The model under review builds one solid part; all positions refer to its coordinate system, in mm. A direction names the side the tool comes from. Coordinates: 2 decimals unless noted, no trailing zeros. Order: outer loops, then holes, each group sorted by start corner. A loop starts at its lowest first (then second) coordinate and runs counter-clockwise, first axis right, second up.
Autodesk Fusion 360 part; units mm, degrees
sketch "Sketch1" plane through (0, 0, 0) normal (0, 1, 0) x (1, 0, 0)
  line L0 (10, 0) -> (76.2, 0)
  line L1 (86.2, 10) -> (86.2, 44.61)
  line L2 (76.2, 54.61) -> (10, 54.61)
  line L3 (0, 44.61) -> (0, 10)
  circle A0 centre (14.6, 51.435) radius 1.6
  circle A1 centre (14.6, 3.175) radius 1.6
  circle A2 centre (80.64, 48.26) radius 1.6
  circle A3 centre (80.64, 6.35) radius 1.6
  arc A4 (0, 10) -> (10, 0) centre (10, 10) ccw
  arc A5 (10, 54.61) -> (0, 44.61) centre (10, 44.61) ccw
  arc A6 (86.2, 44.61) -> (76.2, 54.61) centre (76.2, 44.61) ccw
  arc A7 (76.2, 0) -> (86.2, 10) centre (76.2, 10) ccw
  dimension "d1" = 86.2
  dimension "d2" = 54.61
  dimension "d3" = 3.2
  dimension "d4" = 14.6
  dimension "d5" = 3.175
  dimension "d6" = 48.26
  dimension "d8" = 41.91
  dimension "d10" = 6.35
  dimension "d11" = 65.9
  dimension "d12" = 66.04
  dimension "d13" = 10
  dimension "d36" = 3.11
extrude "Extrude1" add sketch "Sketch1" along normal blind 1.6
sketch "Sketch2" plane through (0, 1.6, 0) normal (0, 1, 0) x (-1, 0, 0)
  circle A0 centre (-14.6, -3.175) radius 1.6
  circle A1 centre (-80.64, -6.35) radius 1.6
  circle A2 centre (-14.6, -51.435) radius 1.6
  circle A3 centre (-80.64, -48.26) radius 1.6
  arc A4 (-76.2, 0) -> (-86.2, -10) centre (-76.2, -10) ccw
  line L0 (-86.2, -10) -> (-86.2, -44.61)
  arc A5 (-86.2, -44.61) -> (-76.2, -54.61) centre (-76.2, -44.61) ccw
  line L1 (-76.2, -54.61) -> (-10, -54.61)
  arc A6 (-10, -54.61) -> (0, -44.61) centre (-10, -44.61) ccw
  line L2 (0, -44.61) -> (0, -10)
  arc A7 (0, -10) -> (-10, 0) centre (-10, -10) ccw
  line L3 (-10, 0) -> (-76.2, 0)
  line L4 (-18.553, -6) -> (-77.553, -6)
  line L5 (-77.553, -6) -> (-77.553, -1)
  line L6 (-77.553, -1) -> (-18.553, -1)
  line L7 (-18.553, -1) -> (-18.553, -6)
  line L8 (-18.553, -53.61) -> (-77.553, -53.61)
  line L9 (-77.553, -53.61) -> (-77.553, -48.61)
  line L10 (-77.553, -48.61) -> (-18.553, -48.61)
  line L11 (-18.553, -48.61) -> (-18.553, -53.61)
  dimension "d16" = 59
  dimension "d17" = 1
  dimension "d18" = 1
  dimension "d19" = 5
extrude "Extrude2" add sketch "Sketch2" along normal blind 8.5 contours L4 L5 L6 L7 | L8 L9 L10 L11
sketch "Sketch3" plane through (0, 1.6, 0) normal (0, 1, 0) x (-1, 0, 0)
  line L0 (-18.553, -1) -> (-18.553, -6)
  line L1 (-18.553, -6) -> (-77.553, -6)
  line L2 (-77.553, -6) -> (-77.553, -1)
  line L3 (-77.553, -1) -> (-18.553, -1)
  line L4 (-18.553, -48.61) -> (-18.553, -53.61)
  line L5 (-18.553, -53.61) -> (-77.553, -53.61)
  line L6 (-77.553, -53.61) -> (-77.553, -48.61)
  line L7 (-77.553, -48.61) -> (-18.553, -48.61)
  circle A0 centre (-14.6, -3.175) radius 1.6
  circle A1 centre (-80.64, -6.35) radius 1.6
  circle A2 centre (-14.6, -51.435) radius 1.6
  circle A3 centre (-80.64, -48.26) radius 1.6
  arc A4 (-76.2, 0) -> (-86.2, -10) centre (-76.2, -10) ccw
  line L8 (-86.2, -10) -> (-86.2, -44.61)
  arc A5 (-86.2, -44.61) -> (-76.2, -54.61) centre (-76.2, -44.61) ccw
  line L9 (-76.2, -54.61) -> (-10, -54.61)
  arc A6 (-10, -54.61) -> (0, -44.61) centre (-10, -44.61) ccw
  line L10 (0, -44.61) -> (0, -10)
  arc A7 (0, -10) -> (-10, 0) centre (-10, -10) ccw
  line L11 (-10, 0) -> (-76.2, 0)
  line L12 (2.5, -37.91) -> (-20.5, -37.91)
  line L13 (-20.5, -37.91) -> (-20.5, -21.61)
  line L14 (-20.5, -21.61) -> (2.5, -21.61)
  line L15 (2.5, -21.61) -> (2.5, -37.91)
  dimension "d22" = 16.3
  dimension "d23" = 16.7
  dimension "d24" = 2.5
extrude "Extrude3" add sketch "Sketch3" along normal blind 13.8 contours L10 L12 L14 L15 | L10 L12 L13 L14
sketch "Sketch4" plane through (0, 1.6, 0) normal (0, 1, 0) x (-1, 0, 0)
  line L0 (-20.5, -21.61) -> (0, -21.61)
  line L1 (0, -21.61) -> (0, -10)
  arc A0 (0, -10) -> (-10, 0) centre (-10, -10) ccw
  line L2 (-10, 0) -> (-76.2, 0)
  arc A1 (-76.2, 0) -> (-86.2, -10) centre (-76.2, -10) ccw
  line L3 (-86.2, -10) -> (-86.2, -44.61)
  arc A2 (-86.2, -44.61) -> (-76.2, -54.61) centre (-76.2, -44.61) ccw
  line L4 (-76.2, -54.61) -> (-10, -54.61)
  arc A3 (-10, -54.61) -> (0, -44.61) centre (-10, -44.61) ccw
  line L5 (0, -44.61) -> (0, -37.91)
  line L6 (0, -37.91) -> (-20.5, -37.91)
  line L7 (-20.5, -37.91) -> (-20.5, -21.61)
  line L8 (-18.553, -1) -> (-18.553, -6)
  line L9 (-18.553, -6) -> (-77.553, -6)
  line L10 (-77.553, -6) -> (-77.553, -1)
  line L11 (-77.553, -1) -> (-18.553, -1)
  line L12 (-18.553, -48.61) -> (-18.553, -53.61)
  line L13 (-18.553, -53.61) -> (-77.553, -53.61)
  line L14 (-77.553, -53.61) -> (-77.553, -48.61)
  line L15 (-77.553, -48.61) -> (-18.553, -48.61)
  circle A4 centre (-14.6, -3.175) radius 1.6
  circle A5 centre (-80.64, -6.35) radius 1.6
  circle A6 centre (-14.6, -51.435) radius 1.6
  circle A7 centre (-80.64, -48.26) radius 1.6
  line L16 (2.5, -14) -> (-11.3258, -14)
  line L17 (-11.3258, -14) -> (-11.3258, -5)
  line L18 (-11.3258, -5) -> (2.5, -5)
  line L19 (2.5, -5) -> (2.5, -14)
  dimension "d27" = 9
  dimension "d28" = 5
extrude "Extrude4" add sketch "Sketch4" along normal blind 11 contours L1 A0 L16 L17 L18 | L1 A0 L16 L18 L19
sketch "Sketch5" plane through (0, 0, 0) normal (0, -1, 0) x (1, 0, 0)
  circle A0 centre (14.6, -3.175) radius 1.6
  circle A1 centre (80.64, -6.35) radius 1.6
  circle A2 centre (14.6, -51.435) radius 1.6
  circle A3 centre (80.64, -48.26) radius 1.6
  arc A4 (86.2, -10) -> (76.2, 0) centre (76.2, -10) ccw
  line L0 (76.2, 0) -> (10, 0)
  arc A5 (10, 0) -> (0, -10) centre (10, -10) ccw
  line L1 (0, -10) -> (0, -44.61)
  arc A6 (0, -44.61) -> (10, -54.61) centre (10, -44.61) ccw
  line L2 (10, -54.61) -> (76.2, -54.61)
  arc A7 (76.2, -54.61) -> (86.2, -44.61) centre (76.2, -44.61) ccw
  line L3 (86.2, -44.61) -> (86.2, -10)
  line L4 (-0.5891, -40.4049) -> (7.6203, -40.4049)
  line L5 (7.6203, -40.4049) -> (7.6203, -46.4306)
  line L6 (7.6203, -46.4306) -> (-0.5891, -46.4306)
  line L7 (-0.5891, -46.4306) -> (-0.5891, -40.4049)
extrude "Extrude5" add sketch "Sketch5" along normal blind 3.9 contours L1 A6 L4 L5 L6 | L1 A6 L4 L6 L7
sketch "Sketch6" plane through (0, 1.6, 0) normal (0, 1, 0) x (-1, 0, 0)
  line L0 (-11.3258, -5) -> (-1.3397, -5)
  arc A0 (-1.3397, -5) -> (-10, 0) centre (-10, -10) ccw
  line L1 (-10, 0) -> (-76.2, 0)
  arc A1 (-76.2, 0) -> (-86.2, -10) centre (-76.2, -10) ccw
  line L2 (-86.2, -10) -> (-86.2, -44.61)
  arc A2 (-86.2, -44.61) -> (-76.2, -54.61) centre (-76.2, -44.61) ccw
  line L3 (-76.2, -54.61) -> (-10, -54.61)
  arc A3 (-10, -54.61) -> (0, -44.61) centre (-10, -44.61) ccw
  line L4 (0, -44.61) -> (0, -37.91)
  line L5 (0, -37.91) -> (-20.5, -37.91)
  line L6 (-20.5, -37.91) -> (-20.5, -21.61)
  line L7 (-20.5, -21.61) -> (0, -21.61)
  line L8 (0, -21.61) -> (0, -14)
  line L9 (0, -14) -> (-11.3258, -14)
  line L10 (-11.3258, -14) -> (-11.3258, -5)
  line L11 (-18.553, -1) -> (-18.553, -6)
  line L12 (-18.553, -6) -> (-77.553, -6)
  line L13 (-77.553, -6) -> (-77.553, -1)
  line L14 (-77.553, -1) -> (-18.553, -1)
  line L15 (-18.553, -48.61) -> (-18.553, -53.61)
  line L16 (-18.553, -53.61) -> (-77.553, -53.61)
  line L17 (-77.553, -53.61) -> (-77.553, -48.61)
  line L18 (-77.553, -48.61) -> (-18.553, -48.61)
  circle A4 centre (-14.6, -3.175) radius 1.6
  circle A5 centre (-80.64, -6.35) radius 1.6
  circle A6 centre (-14.6, -51.435) radius 1.6
  circle A7 centre (-80.64, -48.26) radius 1.6
  line L19 (-44, -35) -> (-62, -35)
  line L20 (-62, -35) -> (-62, -17)
  line L21 (-62, -17) -> (-44, -17)
  line L22 (-44, -17) -> (-44, -35)
  dimension "d33" = 18
extrude "Extrude6" add sketch "Sketch6" along normal blind 2 contours L19 L20 L21 L22
(1) We need section D-D, the plane x = 48. Write out the cut boundary in (y, z).
A:
outline: (0, -54.61) - (1.6, -54.61) - (1.6, -53.61) - (10.1, -53.61) - (10.1, -48.61) - (1.6, -48.61) - (1.6, -35) - (3.6, -35) - (3.6, -17) - (1.6, -17) - (1.6, -6) - (10.1, -6) - (10.1, -1) - (1.6, -1) - (1.6, 0) - (0, 0) - close
(2) Machinability: for faces 5 (the face through (81.5, 0.79, -46.91)), 6 (the face through (18.553, 6, -51)), 7 (the face through (4, -2, -46.431)), which of the approach directions +Z, -Z, +X, -X, +Y, -Y give a long, thin tool a straight path to every point of the face, cutting with its end or side? Answer none if there is none.
A:
face 5: +Y, -Y
face 6: -Z, -X, +Y
face 7: -Z, +X, -X, -Y
(3) We need section C-C, the plane z = -19. Write out the cut boundary in (x, y), and give its area (3 significant figures).
A:
outline: (0, 0) - (86.2, 0) - (86.2, 1.6) - (62, 1.6) - (62, 3.6) - (44, 3.6) - (44, 1.6) - (0, 1.6) - close
area: 174 mm2
(4) Draft analysis for pull direction Z (two halves, no side actions). For faces 1 (the face through (0, 1, -28)), 2 (the face through (44, 3, -26)), 3 (the face through (53, 3, -35)), 4 (the face through (48, 6, -53.61)), state which applies: released by +Z, released by -Z, zero draft, split by the parting line, or undercut.
A:
face 1: zero draft
face 2: undercut
face 3: undercut
face 4: released by -Z
(5) We need section A-A, the plane x = 14.6. Write out the cut boundary in (y, z) (3 decimals).
A:
outline: (0, -54.61) - (1.6, -54.61) - (1.6, -53.035) - (0, -53.035) - close; (0, -49.835) - (1.6, -49.835) - (1.6, -37.91) - (15.4, -37.91) - (15.4, -21.61) - (1.6, -21.61) - (1.6, -4.775) - (0, -4.775) - close; (0, -1.575) - (1.6, -1.575) - (1.6, 0) - (0, 0) - close
(6) Wall thickness on probe 1 along Z at (x, y) = (14.6, 0.65) (3 decimals); probe 2 along Z at (x, y) = (80.64, 0.7); probe 3 along Z at (x, y) = (37.5, 6.75): over which ranges is each line inside the solid? List them lowest first.
A:
probe 1: z = -54.61 to -53.035, -49.835 to -4.775, -1.575 to 0
probe 2: z = -53.57 to -49.86, -46.66 to -7.95, -4.75 to -1.04
probe 3: z = -53.61 to -48.61, -6 to -1
(7) We need section B-B, the plane y = 6.25. Write out the cut boundary in (x, z).
A:
outline: (-2.5, -37.91) - (20.5, -37.91) - (20.5, -21.61) - (-2.5, -21.61) - close; (-2.5, -14) - (11.33, -14) - (11.33, -5) - (-2.5, -5) - close; (18.55, -53.61) - (77.55, -53.61) - (77.55, -48.61) - (18.55, -48.61) - close; (18.55, -6) - (77.55, -6) - (77.55, -1) - (18.55, -1) - close
(8) For pin 1 Ø1.2 at (x, y) = (2, -2) entering from -Z; pin 2 Ø4 at (x, y) = (54.5, 4.5) entering from -Z; pin 3 Ø5 at (y, z) = (-1.5, -15) entering from -X; pin 4 Ø7 at (x, y) = (52, 4.5) entering from +Z, all flat-tipped, find the tip position at first contact; note any pin that passes through.
A:
pin 1: stops at z = -46.43
pin 2: stops at z = -53.61
pin 3: stops at x = 0
pin 4: stops at z = 0
